For this review, use the dimensioned drawing (mm, ordinates from the lowest corner) and the shaded views. A direction names the side the tool comes from. Coordinates: 2 decimals unless noted, no trailing zeros. Loops run counter-clockwise (first coordinate to the right, second up) from the corner with the lowest first, then second, coordinate; pieces in that order, holes last. Notation, with made-up numbers: (75.5, 67) - (89.5, 67) arc R16 ccw to (89.5, 82) - close; hole circle Ø5 at (-5, 59.5). An arc over 180 degrees is marked (long way). Use a Markdown table: item, result. Add a question column.
1) Clearance check with flat-ended pins moving along their axes: pin 1 (10 mm diameter, centred on x = 43, z = 106.5, fed in from +Y); pin 2 (15.5 mm diameter, centred on x = 60.5, y = 52, fed in from +Z). State where each tip first meets the part, or that it passes through.
2) Add section C-C, the plane x = 50. Give the boundary of the cut face in (y, z), and give its area (4 significant figures).
3) Add section D-D, the plane y = 6. Give the boundary of the cut face in (x, z).
4) The part is to be moulded in two halves that separate along X. For the marked faces 3, 4 and 5, say which applies: pulls with the +X half, pulls with the -X half, needs draft (parallel to the pull), parting line crosses it, or undercut.
5) To check wall thickness, follow L1, parallel to Y at x = 50, z = 118; L2, parallel to Z at x = 50, y = 79.5; L3, parallel to Z at x = 31, y = 91. State the ranges of each line that lie inside material, in increasing order. Write a range as [from, to].
6) Add section A-A, the plane z = 50. Give the boundary of the cut face in (x, y).
7) Add section B-B, the plane y = 50. Give the boundary of the cut face in (x, z).
8) For the marked faces 1 and 2, list the 3-axis set-ups (+Z, -Z, +X, -X, +Y, -Y) from which the entire face can be reached by the end or side of a thin tool; tool diameter is ignored.
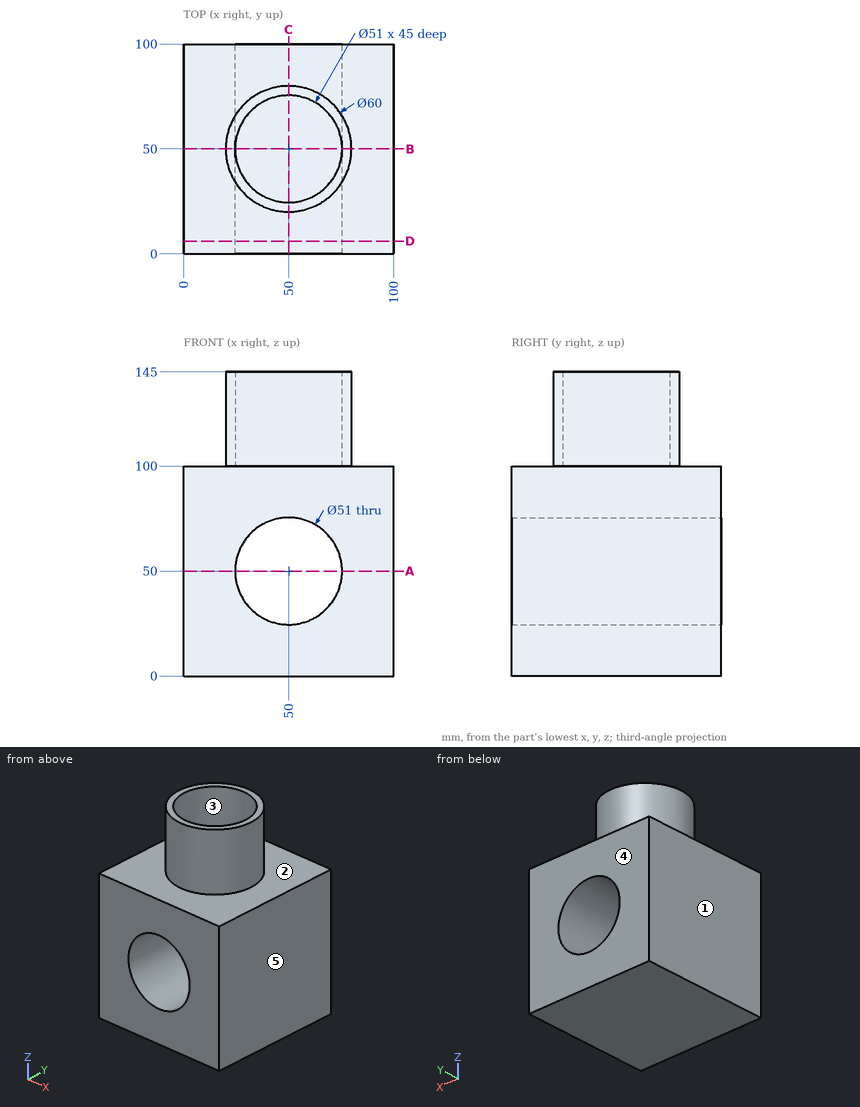
From the geometry:
| question | item | result |
|---|---|---|
| 1 | pin 1 | stops at y = 79.93 |
| 1 | pin 2 | stops at z = 100 |
| 2 | outline | (0, 0) - (100, 0) - (100, 24.5) - (0, 24.5) - close; (0, 75.5) - (100, 75.5) - (100, 100) - (80, 100) - (80, 145) - (75.5, 145) - (75.5, 100) - (24.5, 100) - (24.5, 145) - (20, 145) - (20, 100) - (0, 100) - close |
| 2 | area | 5,305 mm^2 |
| 3 | outline | (0, 0) - (100, 0) - (100, 100) - (0, 100) - close; hole circle Ø51 at (50, 50) |
| 4 | face 3 | undercut |
| 4 | face 4 | needs draft |
| 4 | face 5 | pulls with the +X half |
| 5 | L1 | y = [20, 24.5], [75.5, 80] |
| 5 | L2 | z = [0, 24.5], [75.5, 145] |
| 5 | L3 | z = [0, 32.99], [67.01, 100] |
| 6 | outline | (0, 0) - (24.5, 0) - (24.5, 100) - (0, 100) - close; (75.5, 0) - (100, 0) - (100, 100) - (75.5, 100) - close |
| 7 | outline | (0, 0) - (100, 0) - (100, 100) - (80, 100) - (80, 145) - (75.5, 145) - (75.5, 100) - (24.5, 100) - (24.5, 145) - (20, 145) - (20, 100) - (0, 100) - close; hole circle Ø51 at (50, 50) |
| 8 | face 1 | +Z, -Z, -X, +Y, -Y |
| 8 | face 2 | +Z |
